For this review, use the dimensioned drawing (mm, ordinates from the lowest corner) and the shaded views. Coordinates: 2 decimals unless noted, no trailing zeros. Loops run counter-clockwise (first coordinate to the right, second up) from the corner with the lowest first, then second, coordinate; pieces in that order, holes last. Notation, with made-up numbers: (51.25, 7.25) - (84.25, 7.25) arc R24 cw to (84.25, 36.25) - close; hole circle Ø4 at (37, -5). An arc over 180 degrees is marked (long way). Use one line per item in the form item = value. Start each with the question number.
(1) Add section B-B (y = 100). State the section outline as (x, z) points.
(2) Clearance check with flat-ended pins moving along their axes: pin 1 Ø16 at (x, y) = (177.5, 97.5) entering from -Z; pin 2 Ø3 at (y, z) = (167, 1) entering from -X; pin 3 Ø3 at (x, z) = (162, 3.5) entering from -Y; pin 4 Ø1.5 at (x, z) = (23.5, 4.5) entering from +Y. State where each tip first meets the part, or that it passes through.
(3) Add section D-D (z = 3). State the section outline as (x, y) points.
(4) For L1, parallel to Y at x = 97.5, z = 3.5; L2, parallel to X at y = 95.5, z = 5.35; L3, parallel to Y at x = 112, z = 4.9, list the stretches that pass through material, from the lowest coordinate up.
(5) Add section A-A (y = 129). State the section outline as (x, z) points, plus the area to 3 significant figures.
(6) Add section C-C (x = 177.5). State the section outline as (y, z) points.
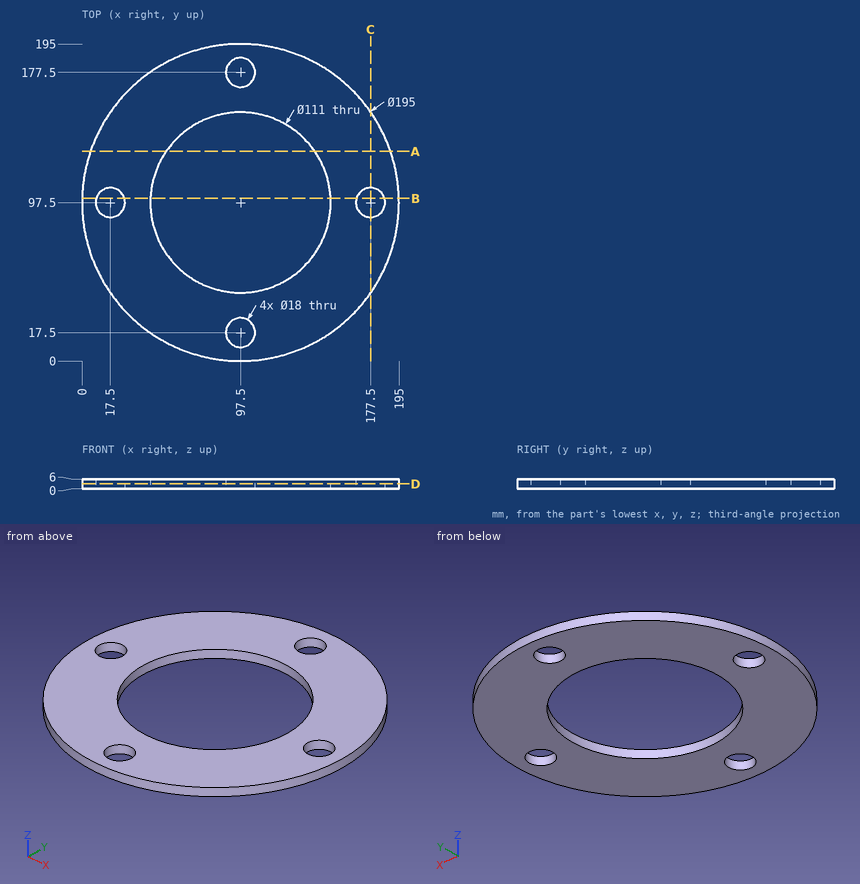
Computed values:
q1.outline = (0.03, 0) - (8.85, 0) - (8.85, 6) - (0.03, 6) - close; (26.15, 0) - (42.06, 0) - (42.06, 6) - (26.15, 6) - close; (152.94, 0) - (168.85, 0) - (168.85, 6) - (152.94, 6) - close; (186.15, 0) - (194.97, 0) - (194.97, 6) - (186.15, 6) - close
q2.pin_1 = through
q2.pin_2 = 27.63
q2.pin_3 = 23.09
q2.pin_4 = 161.85
q3.outline = circle Ø195 at (97.5, 97.5); hole circle Ø18 at (17.5, 97.5); hole circle Ø111 at (97.5, 97.5); hole circle Ø18 at (97.5, 17.5); hole circle Ø18 at (97.5, 177.5); hole circle Ø18 at (177.5, 97.5)
q4.L1 = 0 to 8.5, 26.5 to 42, 153 to 168.5, 186.5 to 195
q4.L2 = 0.02 to 8.73, 26.27 to 42.04, 152.96 to 168.73, 186.27 to 194.98
q4.L3 = 1.08 to 43.93, 151.07 to 193.92
q5.outline = (5.23, 0) - (51.81, 0) - (51.81, 6) - (5.23, 6) - close; (143.19, 0) - (189.77, 0) - (189.77, 6) - (143.19, 6) - close
q5.area = 559 mm^2
q6.outline = (41.77, 0) - (88.5, 0) - (88.5, 6) - (41.77, 6) - close; (106.5, 0) - (153.23, 0) - (153.23, 6) - (106.5, 6) - close
